Read the model definition and answer for the solid it produces. Units are mm, in the model's axes. A direction names the side the tool comes from. Coordinates: 2 decimals unless noted, no trailing zeros. Order: outer loops, then holes, each group sorted by start corner. A loop starts at its lowest first (then second) coordinate and runs counter-clockwise, first axis right, second up. Notation, with made-up numbers: (53.5, -21) - (81.5, -21) arc R14 ccw to (81.5, -5) - close; hole circle Ø7 at (76.5, 85.25). An arc over 180 degrees is marked (long way). Answer as a JSON object with one key per item and string values. Group by question number.
from build123d import *

# Parameters (mm, degrees)
F0_R     = 7.62
F1_DEPTH = 30.734
F2_R     = 2.54
F4_DEPTH = 10.16


with BuildPart() as f1:
    # F0 (on Top) → F1 (new body)
    with BuildSketch(Plane.XY):
        Circle(F0_R)
    extrude(amount=F1_DEPTH)

    # F2
    f2_edges = [f1.edges().sort_by_distance(p)[0] for p in [
        (-7.62, 0, 30.734),
    ]]
    fillet(f2_edges, radius=F2_R)

    # F3 (on Top) → F4 (cut)
    with BuildSketch(Plane.XY):
        Polygon((2.346351, 4.064), (-2.346351, 4.064), (-4.692703, 0), (-2.346351, -4.064), (2.346351, -4.064), (4.692703, 0), align=None)
    extrude(amount=F4_DEPTH, mode=Mode.SUBTRACT)


solid = f1.part
1. Straight lines are drawn through the part: L1, parallel to Z at x = 3.5, y = -1.5; L2, parallel to X at y = -6, z = 27.5; L3, parallel to Y at x = -1.75, z = 2.5. For each, find the intervals that lie inside material, in ascending order.
2. A cutting plane is placed at B-B on x = 0. Write down the section's boundary in (y, z), and give its area (3 significant figures).
3. Given pin 1 (1 mm diameter, centred on x = -2, y = -2, fed in from -Z); pin 2 (1.5 mm diameter, centred on y = -1.5, z = 12.5, fed in from +X); pin 3 (1.5 mm diameter, centred on y = -3, z = 4, fed in from -X), each flat-ended and moving along its own axis, determine where each tip first touches the part or whether it passes through.
4. For faces 1 (the flat face through (3.3, -3.3, 0)), 2 (the flat face through (0, 4.064, 5)), determine the directions among +Z, -Z, +X, -X, +Y, -Y from which every point of the face is accessible in a straight line to the end or side of a thin tool.
5. A cutting plane is placed at C-C on z = 26.5. Write down the section's boundary in (x, y), and give its area (3 significant figures).
6. For a pull along Y with two mould halves and no side action, classify faces 3 (the flat face through (-3.503, 2.06, 5.009)), 4 (the flat face through (0, 0, 10.16)), 5 (the cylindrical face through (-1.65, -7.44, 13.9)), 6 (the flat face through (0, 0, 30.734)) as pulls with the +Y half, pulls with the -Y half, needs draft (parallel to the pull), parting line crosses it, or undercut.
7. A cutting plane is placed at A-A on z = 3.5. Write down the section's boundary in (x, y), and give its area (3 significant figures).
Derived:
{
 "1": {"L1": "z = 10.16 to 30.73", "L2": "x = -4.7 to 4.7", "L3": "y = -7.42 to -4.06, 4.06 to 7.42"},
 "2": {"outline": "(-7.62, 0) - (-4.06, 0) - (-4.06, 10.16) - (4.06, 10.16) - (4.06, 0) - (7.62, 0) - (7.62, 28.19) arc R2.54 ccw to (5.08, 30.73) - (-5.08, 30.73) arc R2.54 ccw to (-7.62, 28.19) - close", "area": "383 mm2"},
 "3": {"pin 1": "stops at z = 10.16", "pin 2": "stops at x = 7.58", "pin 3": "stops at x = -7.28"},
 "4": {"face 1": "-Z, +X, -X, +Y, -Y", "face 2": "-Z"},
 "5": {"outline": "circle Ø15.24 at (0, 0)", "area": "182 mm2"},
 "6": {"face 3": "undercut", "face 4": "undercut", "face 5": "parting line crosses it", "face 6": "needs draft"},
 "7": {"outline": "circle Ø15.24 at (0, 0); hole (-4.69, 0) - (-2.35, -4.06) - (2.35, -4.06) - (4.69, 0) - (2.35, 4.06) - (-2.35, 4.06) - close", "area": "125 mm2"}
}
